```python
from build123d import *

# Parameters (mm, degrees)
BOSS_EXTRU_1_DEPTH = 8


with BuildPart() as part:
    # Esquisse4 → Boss.-Extru.1 (new body)
    with BuildSketch(Plane(origin=(0, 0, 0), x_dir=(1, 0, 0), z_dir=(0, 1, 0))):
        with BuildLine():
            ThreePointArc((-1.341955193, -10.413892464), (-1.552117835, -9.051281003), (-1.997724586, -7.746553845))
            ThreePointArc((-1.997724586, -7.746553845), (-7.802132308, -1.768256613), (-5.142300877, 6.128355545))
            ThreePointArc((-5.142300877, 6.128355545), (-5.499269902, 7.46058208), (-6.749269902, 8.043466653))
            ThreePointArc((-6.749269902, 8.043466653), (-10.5, 0), (-6.749269902, -8.043466653))
            ThreePointArc((-6.749269902, -8.043466653), (-4.215650663, -9.616563289), (-1.341955193, -10.413892464))
        make_face()
        with BuildLine():
            ThreePointArc((6.749269902, 8.043466653), (5.499269902, 7.46058208), (5.142300877, 6.128355545))
            ThreePointArc((5.142300877, 6.128355545), (7.11339354, -3.660550825), (-1.997724586, -7.746553845))
            ThreePointArc((-1.997724586, -7.746553845), (-1.552117835, -9.051281003), (-1.341955193, -10.413892464))
            ThreePointArc((-1.341955193, -10.413892464), (9.616563289, -4.215650663), (6.749269902, 8.043466653))
        make_face()
        with BuildLine():
            ThreePointArc((-6.389571855, -18.255279028), (-2.573158, -15.166655065), (-1.341955193, -10.413892464))
            ThreePointArc((-1.341955193, -10.413892464), (-4.215650663, -9.616563289), (-6.749269902, -8.043466653))
            ThreePointArc((-6.749269902, -8.043466653), (-5.459487684, -11.551992452), (-7.834566209, -14.438563679))
            ThreePointArc((-7.834566209, -14.438563679), (-9.020426707, -17.06941853), (-6.389571855, -18.255279028))
        make_face()
    boss_extru_1 = extrude(amount=BOSS_EXTRU_1_DEPTH)

    # Symétrie1: Boss.-Extru.1 across plane
    add(boss_extru_1.mirror(Plane(origin=(0, 0, 0), x_dir=(0, 0, 1), z_dir=(1, 0, 0))))


solid = part.part
```
Input: part model. Units: mm. Frame: model coordinates. Coordinates: 2 decimals unless noted, no trailing zeros. Write each loop counter-clockwise with the first axis right and the second up, starting at its lowest first coordinate (ties: lowest second). Pieces come first, ordered by that corner, then holes. Notation, with made-up numbers: (10, -15.75) -> (53, -15.75) arc R28 ccw to (53, 12.25) -> close; hole circle Ø6 at (-23.5, 19.25). An arc over 180 degrees is marked (long way). Write each question's results on one line, items separated by ' | '.
Item 1: Mould query, pull axis Z, two halves, no side actions, for faces 1 (the cylindrical face through (-5.45, 3.94, 11.5)), 2 (the flat face through (2, 8, 9)). Classes: +Z half, -Z half, draft (parallel to the pull), parting line (faces both ways), or undercut.
Conclusion:
face 1: undercut | face 2: draft
Item 2: Pin query (flat end, axial travel): pin 1 Ø3 at (x, z) = (7, 2) entering from +Y; pin 2 Ø1.5 at (y, z) = (6, 7.5) entering from -X; pin 3 Ø4 at (x, y) = (1.5, 4.5) entering from +Z; pin 4 Ø3 at (y, z) = (6, 10.5) entering from +X. Return the tip coordinate at first contact, or that it passes through.
Conclusion:
pin 1: stops at y = 8 | pin 2: stops at x = -8.04 | pin 3: stops at z = 16.34 | pin 4: stops at x = 5.94
Item 3: Section query B-B on z = 0. Return loops of the section in (x, y), plus the area to 3 significant figures.
Conclusion:
outline: (-10.5, 0) -> (-8, 0) -> (-8, 8) -> (-10.5, 8) -> close; (8, 0) -> (10.5, 0) -> (10.5, 8) -> (8, 8) -> close | area: 40.0 mm^2
Item 4: Section query D-D on y = 4.75. Return loops of the section in (x, z).
Conclusion:
outline: (-7.83, 14.44) arc R3.76 cw to (-6.75, 8.04) arc R10.5 ccw to (-6.75, -8.04) arc R1.63 ccw to (-5.14, -6.13) arc R8 cw (long way) to (5.14, -6.13) arc R1.63 ccw to (6.75, -8.04) arc R10.5 ccw to (6.75, 8.04) arc R3.76 cw to (7.83, 14.44) arc R2.04 ccw to (6.39, 18.26) arc R7.84 ccw to (1.34, 10.41) arc R10.5 ccw to (-1.34, 10.41) arc R7.84 ccw to (-6.39, 18.26) arc R2.04 ccw to start
Item 5: Section query A-A on x = 7.5. Return loops of the section in (y, z).
Conclusion:
outline: (0, -7.35) -> (8, -7.35) -> (8, -2.78) -> (0, -2.78) -> close; (0, 2.78) -> (8, 2.78) -> (8, 7.35) -> (0, 7.35) -> close; (0, 14.29) -> (8, 14.29) -> (8, 18.35) -> (0, 18.35) -> close
Item 6: Material intervals for probe 1 along Z at (x, y) = (6, 7); probe 2 along Z at (x, y) = (6.25, 7); probe 3 along X at (y, z) = (0.5, -5.5), sorted ascending.
Conclusion:
probe 1: z = -7.86 to -5.29, 5.29 to 8.9, 12.95 to 18.1 | probe 2: z = -7.97 to -4.99, 4.99 to 8.55, 13.3 to 18.2 | probe 3: x = -8.94 to -5.81, 5.81 to 8.94
Item 7: Section query C-C on x = -8.75. Return loops of the section in (y, z).
Conclusion:
outline: (0, -5.8) -> (8, -5.8) -> (8, 5.8) -> (0, 5.8) -> close; (0, 15.13) -> (8, 15.13) -> (8, 17.56) -> (0, 17.56) -> close
